from build123d import *

# Parameters (mm, degrees)
SKETCH1_W           = 35
SKETCH1_H           = 55
BOSS_EXTRUDE1_DEPTH = 0.775
SKETCH2_R           = 1.75
CUT_EXTRUDE1_DEPTH  = 5


with BuildPart() as part:
    # Sketch1 → Boss-Extrude1 (new, symmetric)
    with BuildSketch(Plane(origin=(0, 0, 0), x_dir=(1, 0, 0), z_dir=(0, 1, 0))):
        Rectangle(SKETCH1_W, SKETCH1_H)
    extrude(amount=BOSS_EXTRUDE1_DEPTH, both=True)

    # Sketch2 → Cut-Extrude1 (cut, symmetric)
    with BuildSketch(Plane(origin=(0, 0, 0), x_dir=(1, 0, 0), z_dir=(0, 1, 0))):
        with Locations(Location((0, 7, 0), (0, 0, 270))):
            Circle(SKETCH2_R)
        with Locations(Location((0, -7, 0), (0, 0, 270))):
            Circle(SKETCH2_R)
    extrude(amount=CUT_EXTRUDE1_DEPTH, both=True, mode=Mode.SUBTRACT)


solid = part.part
Can you work these out from the model? Positions are in its coordinate system, mm. Round coordinates to 2 decimals unless told otherwise and drop trailing zeros. Order: outer loops, then holes, each group sorted by start corner. A loop starts at its lowest first (then second) coordinate and runs counter-clockwise, first axis right, second up. Notation, with made-up numbers: M -23,-37.5 L 14,-37.5 A3 ccw 14,-32.5 Z; hole C -40,-32.5 d2. An arc over 180 degrees is marked long. Use a Markdown table: item, result.
1) Imagine slicing it at A-A (z = -7). List the corners of the cut face in (x, y) for me (3 decimals), then the cut area to 3 significant figures.
Geometry says:
| item | result |
|---|---|
| outline | M -17.5,-0.775 L -1.75,-0.775 L -1.75,0.775 L -17.5,0.775 Z; M 1.75,-0.775 L 17.5,-0.775 L 17.5,0.775 L 1.75,0.775 Z |
| area | 48.8 mm² |
2) If I drill on line 1 along X through (y, z) = (0.05, 7); line 2 along Z through (x, y) = (1, 0.5); line 3 along X through (y, z) = (-0.4, 5.5), over which ranges is the centre line in solid material (lowest first)?
Geometry says:
| item | result |
|---|---|
| line 1 | x = -17.5 to -1.75, 1.75 to 17.5 |
| line 2 | z = -27.5 to -8.44, -5.56 to 5.56, 8.44 to 27.5 |
| line 3 | x = -17.5 to -0.9, 0.9 to 17.5 |
3) If we mould it in two halves opening along X, with no side actions, what happens to faces 1 (the face through (17.5, 0, 0)), 2 (the face through (0.526, 0.011, 8.669)), 3 (the face through (0, 0, 27.5))? For each: +X half, -X half, draft (parallel to the pull), parting line (faces both ways), or undercut.
Geometry says:
| item | result |
|---|---|
| face 1 | +X half |
| face 2 | undercut |
| face 3 | draft |
4) Imagine slicing it at B-B (x = 0). List the corners of the cut face in (y, z) for me (3 decimals).
Geometry says:
| item | result |
|---|---|
| outline | M -0.775,-27.5 L 0.775,-27.5 L 0.775,-8.75 L -0.775,-8.75 Z; M -0.775,-5.25 L 0.775,-5.25 L 0.775,5.25 L -0.775,5.25 Z; M -0.775,8.75 L 0.775,8.75 L 0.775,27.5 L -0.775,27.5 Z |
5) I'm going to push a flat-ended pin straight in: P1, Ø3, axis at x = 0, z = -7, coming from the +Y side. Where does the tip first touch, or does it pass through?
Geometry says:
| item | result |
|---|---|
| P1 | passes through |
